For this review, use the dimensioned drawing (mm, ordinates from the lowest corner) and the shaded views. Give positions to 0.01 mm unless a question says otherwise; leave off trailing zeros. Order: outer loops, then holes, each group sorted by start corner. A loop starts at its lowest first (then second) coordinate and runs counter-clockwise, first axis right, second up.
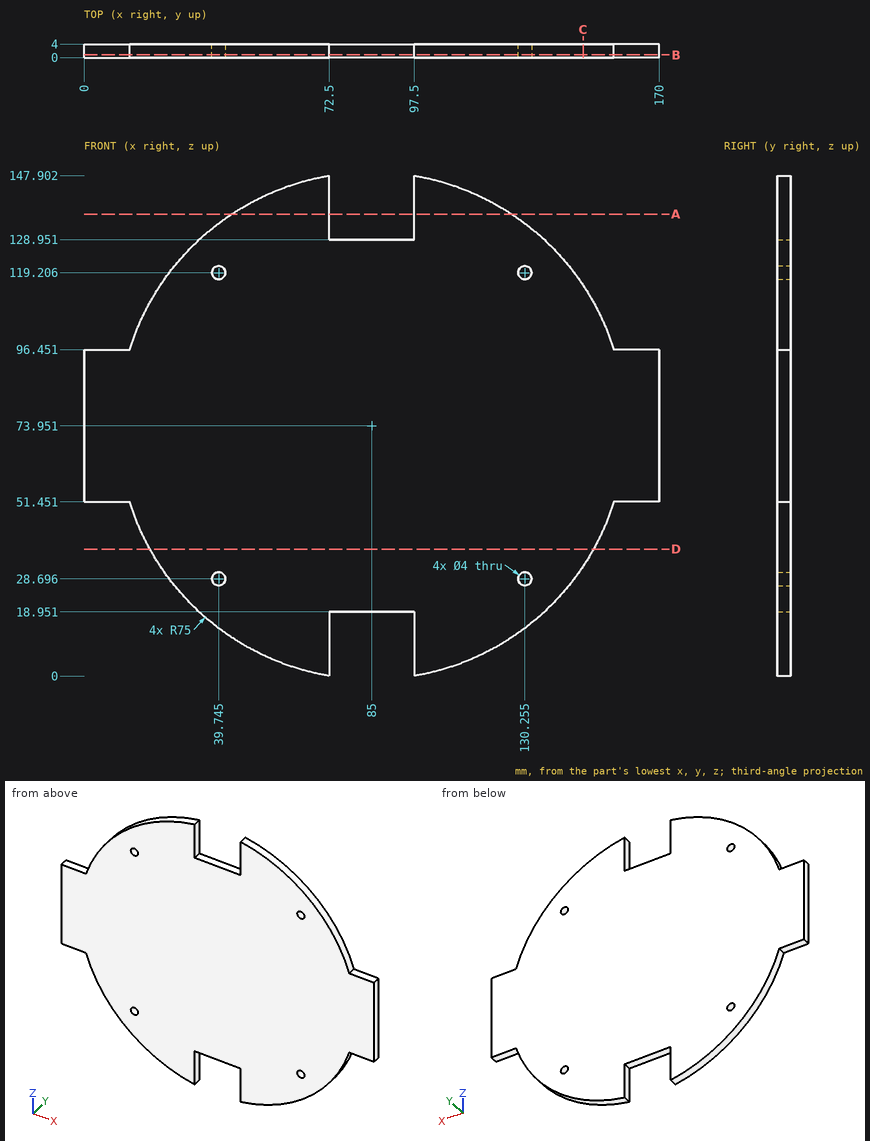
1. Take a section at C-C (x = 147.5). Write out the cut boundary in (y, z), and give its area (3 significant figures).
2. Take a section at D-D (z = 37.5). Write out the cut boundary in (x, y).
3. Take a section at B-B (y = 0.8). Write out the cut boundary in (x, z) (1 decimal), and give its area (3 significant figures).
4. Take a section at A-A (z = 136.5). Write out the cut boundary in (x, y), and give its area (3 significant figures).
5. To check wall thickness, follow line 1 (X direction, y = 2.25, z = 27.5); line 2 (X direction, y = 0.3, z = 119.5) (1 decimal); line 3 (Z direction, x = 76, y = 3.2). State the ranges of each line that lie inside material, in increasing order.
6. Insertion check: pin 1 (2 mm diameter, centred on y = 0.5, z = 42, fed in from -X); pin 2 (1.2 mm diameter, centred on y = 2.5, z = 136, fed in from +X); pin 3 (2.5 mm diameter, centred on x = 130.25, z = 28.7, fed in from -Y); pin 4 (2 mm diameter, centred on x = 165.5, y = 2.5, fed in from +Z). Each pin has a flat end and moves straight along its axis. Give the tip position at first contact, or say it passes through.
Answer:
1. outline: (0, 32.49) - (4, 32.49) - (4, 115.41) - (0, 115.41) - close
1. area: 332 mm2
2. outline: (19.45, 0) - (150.55, 0) - (150.55, 4) - (19.45, 4) - close
3. outline: (0, 51.5) - (13.5, 51.5) arc R75 ccw to (72.5, 0) - (72.5, 19) - (97.5, 19) - (97.5, 0) arc R75 ccw to (156.5, 51.5) - (170, 51.5) - (170, 96.5) - (156.5, 96.5) arc R75 ccw to (97.5, 147.9) - (97.5, 129) - (72.5, 129) - (72.5, 147.9) arc R75 ccw to (13.5, 96.5) - (0, 96.5) - close; hole circle Ø4 at (39.7, 28.7); hole circle Ø4 at (39.7, 119.2); hole circle Ø4 at (130.3, 28.7); hole circle Ø4 at (130.3, 119.2)
3. area: 17,600 mm2
4. outline: (43.62, 0) - (72.5, 0) - (72.5, 4) - (43.62, 4) - close; (97.5, 0) - (126.38, 0) - (126.38, 4) - (97.5, 4) - close
4. area: 231 mm2
5. line 1: x = 26.12 to 38.14, 41.35 to 128.65, 131.86 to 143.88
5. line 2: x = 25.4 to 37.8, 41.7 to 128.3, 132.2 to 144.6
5. line 3: z = 18.95 to 128.95
6. pin 1: stops at x = 16.68
6. pin 2: stops at x = 128
6. pin 3: passes through
6. pin 4: stops at z = 96.45
